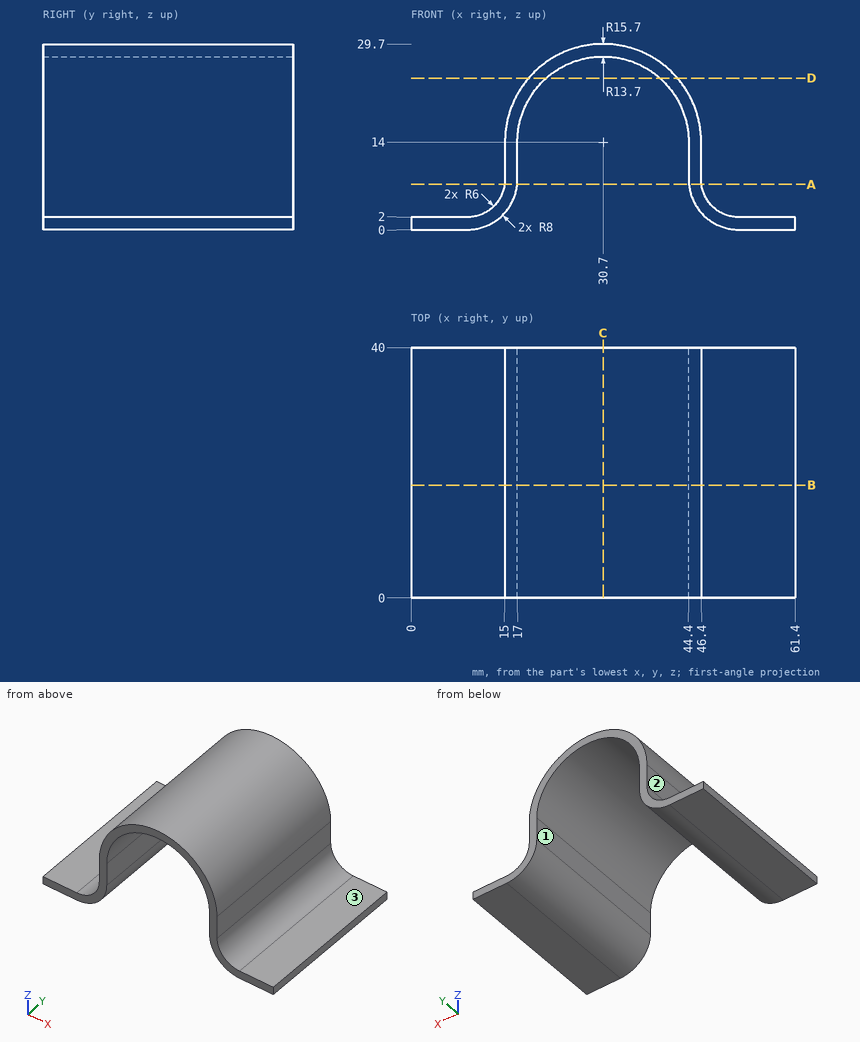
Print and shaded views of the part. All mm, measured from the part's lowest x, y and z. A direction names the side the tool comes from. Coordinates: 2 decimals unless noted, no trailing zeros. Order: outer loops, then holes, each group sorted by start corner. A loop starts at its lowest first (then second) coordinate and runs counter-clockwise, first axis right, second up. Notation, with made-up numbers: (36, 25.25) -> (69, 25.25) arc R22 cw to (69, 56.25) -> close; hole circle Ø1 at (19, 30). An arc over 180 degrees is marked (long way). Use one line per item in the form item = value. Start each with the question number.
1) Band-saw the part on A-A on z = 7.25. Give the cut face in (x, y), then the cut area to 3 significant figures.
2) Drill centre lines: L1, parallel to X at y = 31.5, z = 13; L2, parallel to Z at x = 52.5, y = 19; L3, parallel to X at y = 31.5, z = 15.5. Where is each one in solid material? Low to high. Write a range as [from, to].
3) Band-saw the part on B-B on y = 18. Give the cut face in (x, z), then the cut area to 3 significant figures.
4) Tool access for the marked faces 1, 2 and 3: list every direction of +Z, -Z, +X, -X, +Y, -Y with a clear straight run to the whole face (end or side of a thin tool).
5) Drop flat-ended pins along their axis: pin 1 (6.5 mm diameter, centred on y = 14.5, z = 11.5, fed in from +X); pin 2 (10 mm diameter, centred on x = 5.5, y = 28, fed in from +Z); pin 3 (5 mm diameter, centred on y = 25.5, z = 10, fed in from -X); pin 4 (6 mm diameter, centred on x = 15, z = 24, fed in from -Y). Give the stop position or say it passes through.
6) Band-saw the part on C-C on x = 30.7. Give the cut face in (y, z), then the cut area to 3 significant figures.
7) Band-saw the part on D-D on z = 24.25. Give the cut face in (x, y).
Entries:
q1.outline = (14.95, 0) -> (16.96, 0) -> (16.96, 40) -> (14.95, 40) -> close; (44.44, 0) -> (46.45, 0) -> (46.45, 40) -> (44.44, 40) -> close
q1.area = 161 mm2
q2.L1 = [15, 17], [44.4, 46.4]
q2.L2 = [0, 2]
q2.L3 = [15.07, 17.08], [44.32, 46.33]
q3.outline = (0, 0) -> (9, 0) arc R8 ccw to (17, 8) -> (17, 14) arc R13.7 cw to (44.4, 14) -> (44.4, 8) arc R8 ccw to (52.4, 0) -> (61.4, 0) -> (61.4, 2) -> (52.4, 2) arc R6 cw to (46.4, 8) -> (46.4, 14) arc R15.7 ccw to (15, 14) -> (15, 8) arc R6 cw to (9, 2) -> (0, 2) -> close
q3.area = 196 mm2
q4.face_1 = -Z, +Y, -Y
q4.face_2 = +Z, -X, +Y, -Y
q4.face_3 = +Z, +X, +Y, -Y
q5.pin_1 = 46.4
q5.pin_2 = 2.19
q5.pin_3 = 14.98
q5.pin_4 = 0
q6.outline = (0, 27.7) -> (40, 27.7) -> (40, 29.7) -> (0, 29.7) -> close
q6.area = 80.0 mm2
q7.outline = (18.81, 0) -> (21.61, 0) -> (21.61, 40) -> (18.81, 40) -> close; (39.79, 0) -> (42.59, 0) -> (42.59, 40) -> (39.79, 40) -> close
